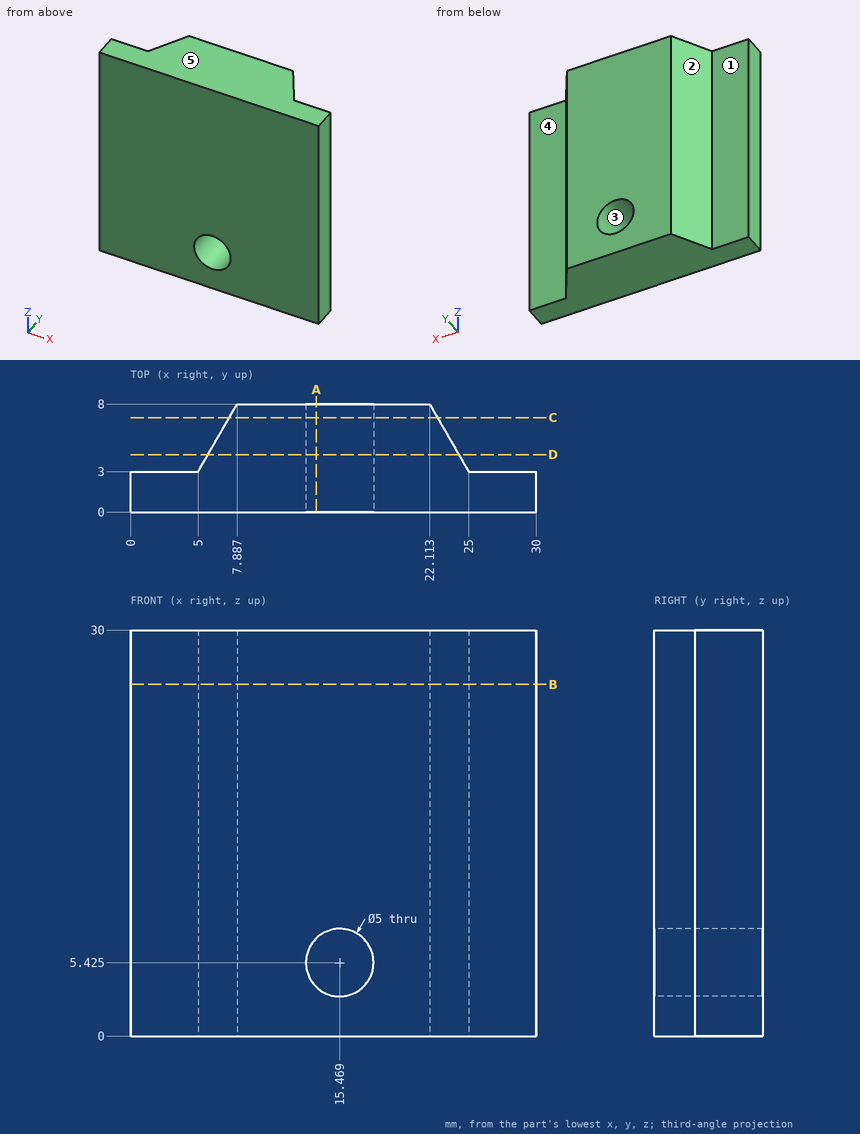
Design review of the part shown in the three views and the two pictorial views. Dimensions are in mm from the part's minimum x, y and z. A direction names the side the tool comes from. Give positions to 0.01 mm unless a question says otherwise; leave off trailing zeros. Write each loop counter-clockwise with the first axis right and the second up, starting at its lowest first coordinate (ties: lowest second). Pieces come first, ordered by that corner, then holes. Notation, with made-up numbers: (39.25, -28.75) - (54.25, -28.75) arc R8 ccw to (54.25, -20.75) - close; hole circle Ø11 at (47.5, 33). An arc over 180 degrees is marked (long way). Return JSON: item names as keys, results as strings. Group by question number.
(1) We need section C-C, the plane y = 7. Give the boundary of the cut face in (x, z) (1 decimal).
(2) We need section D-D, the plane y = 4.25. Give the boundary of the cut face in (x, z) (1 decimal), then the cut area to 3 significant figures.
(3) Insertion check: pin 1 (4 mm diameter, centred on x = 15.47, z = 5.43, fed in from -Y); pin 2 (4 mm diameter, centred on x = 28, z = 12, fed in from +Y); pin 3 (5.5 mm diameter, centred on x = 3, z = 8, fed in from +Y). Each pin has a flat end and moves straight along its axis. Give the tip position at first contact, or say it passes through.
(4) To check wall thickness, follow probe 1 along Z at (x, y) = (15.5, 0.5) (1 decimal); probe 2 along X at (y, z) = (3.75, 5.5); probe 3 along X at (y, z) = (5, 5.5) (1 decimal). State the ranges of each line that lie inside material, in increasing order.
(5) Mouldability with a two-part tool opening along X and no side actions: class the marked faces 1, 2 and 3 as +X half, -X half, draft (parallel to the pull), parting line (faces both ways), or undercut.
(6) We need section B-B, the plane z = 26. Give the boundary of the cut face in (x, y), then the cut area to 3 significant figures.
(7) Machinability: for the marked faces 4 and 5, which of the approach directions +Z, -Z, +X, -X, +Y, -Y give a long, thin tool a straight path to every point of the face, cutting with its end or side? Answer none if there is none.
(8) We need section A-A, the plane x = 13.75. Give the boundary of the cut face in (y, z), then the cut area to 3 significant figures.
Reported:
{
 "1": {"outline": "(7.3, 0) - (22.7, 0) - (22.7, 30) - (7.3, 30) - close; hole circle Ø5 at (15.5, 5.4)"},
 "2": {"outline": "(5.7, 0) - (24.3, 0) - (24.3, 30) - (5.7, 30) - close; hole circle Ø5 at (15.5, 5.4)", "area": "537 mm2"},
 "3": {"pin 1": "passes through", "pin 2": "stops at y = 3", "pin 3": "stops at y = 4.3"},
 "4": {"probe 1": "z = 0 to 2.9, 7.9 to 30", "probe 2": "x = 5.43 to 12.97, 17.97 to 24.57", "probe 3": "x = 6.2 to 13, 18 to 23.8"},
 "5": {"face 1": "draft", "face 2": "-X half", "face 3": "undercut"},
 "6": {"outline": "(0, 0) - (30, 0) - (30, 3) - (25, 3) - (22.11, 8) - (7.89, 8) - (5, 3) - (0, 3) - close", "area": "176 mm2"},
 "7": {"face 4": "+Z, -Z, +X, +Y", "face 5": "+Z, +X, -X, +Y, -Y"},
 "8": {"outline": "(0, 0) - (8, 0) - (8, 3.61) - (0, 3.61) - close; (0, 7.24) - (8, 7.24) - (8, 30) - (0, 30) - close", "area": "211 mm2"}
}
